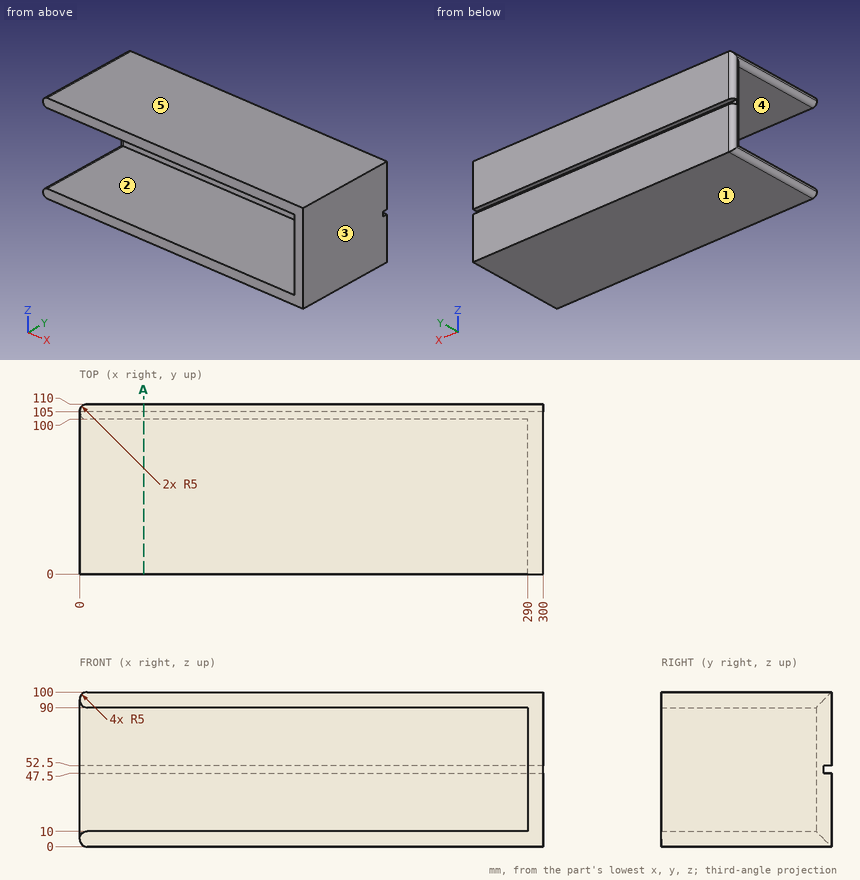
Answer from the drawing. Dimensions are ordinates in mm from the lowest x, y and z of the part. A direction names the side the tool comes from. Give positions to 0.01 mm unless a question says otherwise; leave off trailing zeros. Loops run counter-clockwise (first coordinate to the right, second up) from the corner with the lowest first, then second, coordinate; pieces in that order, holes last. Notation, with made-up numbers: (-28, -36) - (-6, -36) arc R22 cw to (-6, 1) - close; hole circle Ø9 at (37.5, -31). An arc over 180 degrees is marked (long way). Write each question's results on one line, items separated by ' | '.
1. Consider probe 1 along Z at (x, y) = (162, 21); probe 2 along X at (y, z) = (65, 50); probe 3 along Y at (x, z) = (168.5, 54). Determine where each line is inside the solid, lowest interval first. Write a range as from..to.
Resolved:
probe 1: z = 0..10, 90..100 | probe 2: x = 290..300 | probe 3: y = 100..110
2. Flat-ended cylindrical pins translate along their axes: P1, Ø1.5, axis at y = 26, z = 45, coming from the -X side; P2, Ø1.5, axis at x = 201, z = 50.5, coming from the +Y side. Find the tip coordinate at first contact, or state that the pin passes through.
Resolved:
P1: stops at x = 290 | P2: stops at y = 105
3. Which of the six approach directions +Z, -Z, +X, -X, +Y, -Y give full straight-line access (tool end or side, diameter ignored) to the marked faces 4 and 5?
Resolved:
face 4: -X, -Y | face 5: +Z, +X, -X, +Y, -Y
4. For a pull along Z with two mould halves and no side action, classify the marked faces 1, 2 and 3 as +Z half, -Z half, draft (parallel to the pull), parting line (faces both ways), or undercut.
Resolved:
face 1: -Z half | face 2: undercut | face 3: draft
5. Find section A-A, the plane x = 41.5. Write down the section's boundary in (y, z), then the cut area to 4 significant figures.
Resolved:
outline: (0, 0) - (110, 0) - (110, 47.5) - (105, 47.5) - (105, 52.5) - (110, 52.5) - (110, 100) - (0, 100) - (0, 90) - (100, 90) - (100, 10) - (0, 10) - close | area: 2,975 mm^2
